Geometry: see drawing. Coordinates: mm, zero at the bounding-box minimum. A direction names the side the tool comes from. Give positions to 0.01 mm unless a question says otherwise; leave off trailing zeros. Loops run counter-clockwise (first coordinate to the right, second up) from the corner with the lowest first, then second, coordinate; pieces in that order, holes last. Notation, with made-up numbers: (-2.5, 71) -> (21.5, 71) arc R14 ccw to (21.5, 86) -> close; hole circle Ø4 at (52.25, -17). An arc over 180 degrees is marked (long way). Use CSV: the item, a comma, the result in double quotes.
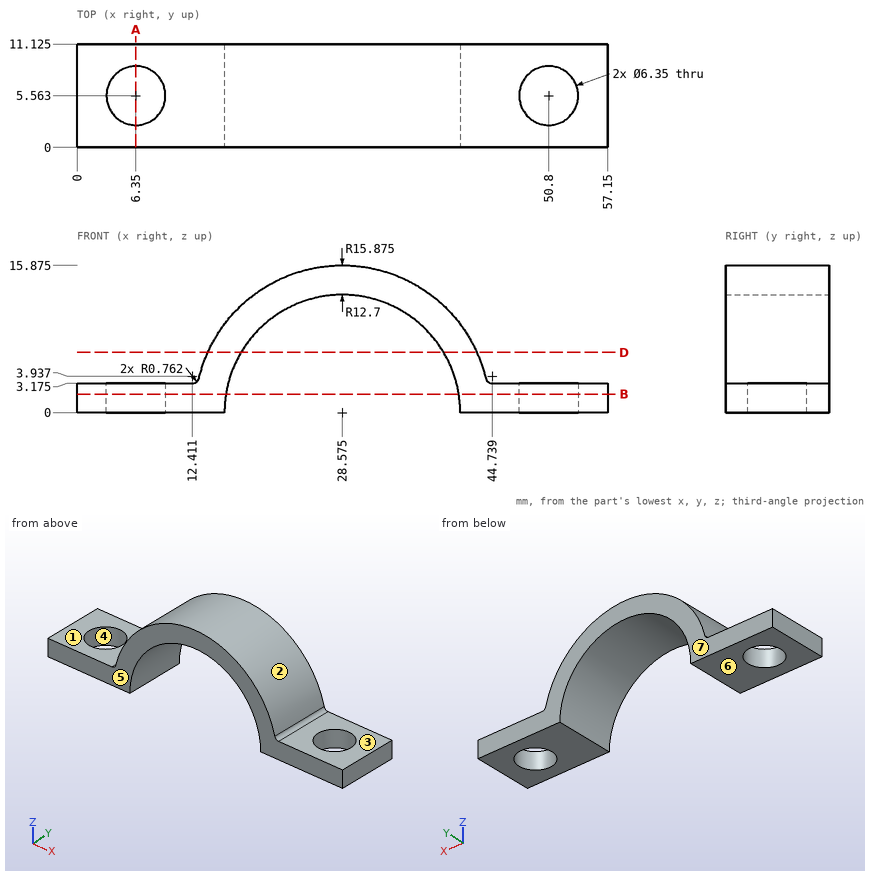
1) Section query A-A (x = 6.35). Return loops of the section in (y, z) (1 decimal).
From the geometry:
outline,"(0, 0) -> (2.4, 0) -> (2.4, 3.2) -> (0, 3.2) -> close; (8.7, 0) -> (11.1, 0) -> (11.1, 3.2) -> (8.7, 3.2) -> close"
2) Section query D-D (z = 6.5). Return loops of the section in (x, y) (1 decimal).
From the geometry:
outline,"(14.1, 0) -> (17.7, 0) -> (17.7, 11.1) -> (14.1, 11.1) -> close; (39.5, 0) -> (43.1, 0) -> (43.1, 11.1) -> (39.5, 11.1) -> close"
3) Reachability of the marked faces 1, 2 and 3 from +Z, -Z, +X, -X, +Y, -Y: full face, straight path, thin tool, end or side. Return the list, or none.
From the geometry:
face 1,"+Z, -X, +Y, -Y"
face 2,"+Z, +Y, -Y"
face 3,"+Z, +X, +Y, -Y"
4) Contact query for flat-ended pins moving along their axis: pin 1 (3.5 mm diameter, centred on x = 49.5, y = 4, fed in from +Z) (3 decimals); pin 2 (5 mm diameter, centred on y = 7.5, z = 11, fed in from +X); pin 3 (2 mm diameter, centred on x = 32, y = 2.5, fed in from +Z). Output: stop coordinate, or through.
From the geometry:
pin 1,"stops at z = 3.175"
pin 2,"stops at x = 41.98"
pin 3,"stops at z = 15.69"
5) Mould query, pull axis Y, two halves, no side actions, for the marked faces 4, 5, 6 and 7. Classes: pulls with the +Y half, pulls with the -Y half, needs draft (parallel to the pull), parting line crosses it, or undercut.
From the geometry:
face 4,"undercut"
face 5,"pulls with the -Y half"
face 6,"needs draft"
face 7,"pulls with the +Y half"
6) Section query B-B (z = 2). Give the number of separate pieces and of enclosed holes in the cut face.
From the geometry:
separate pieces,"2"
enclosed holes,"2"
7) Ray query, line 1 (Y direction, x = 6.35, z = 0.8) (1 decimal); line 2 (X direction, y = 4.5, z = 8.5) (1 decimal); line 3 (X direction, y = 7, z = 5). Return the intervals inside material, ascending.
From the geometry:
line 1,"y = 0 to 2.4, 8.7 to 11.1"
line 2,"x = 15.2 to 19.1, 38 to 42"
line 3,"x = 13.51 to 16.9, 40.25 to 43.64"
